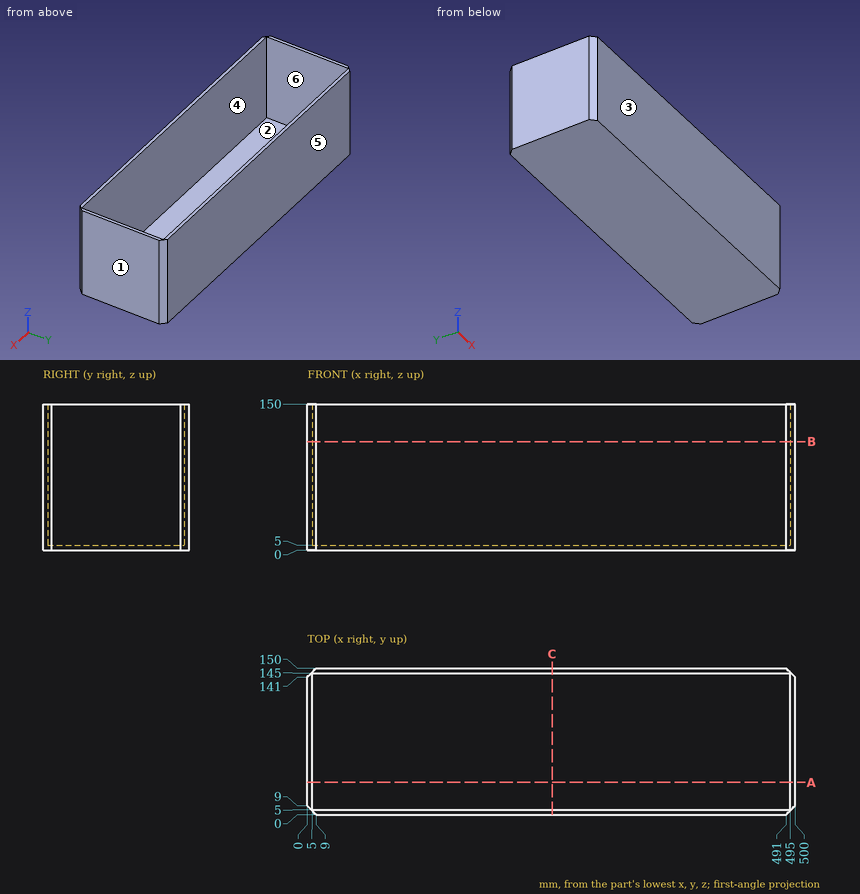
For this review, use the dimensioned drawing (mm, ordinates from the lowest corner) and the shaded views. A direction names the side the tool comes from. Give positions to 0.01 mm unless a question says otherwise; leave off trailing zeros. Order: outer loops, then holes, each group sorted by start corner. A loop starts at its lowest first (then second) coordinate and runs counter-clockwise, first axis right, second up. Notation, with made-up numbers: (-21, 7.25) - (35, 7.25) arc R8 ccw to (35, 13.25) - close; hole circle Ø9 at (-24, 28). An arc over 180 degrees is marked (long way). Use CSV: the item, a comma, the result in double quotes. Start each with the question number.
Q1. To check wall thickness, follow line 1 along Y through (x, z) = (461, 96); line 2 along X through (y, z) = (121, 10); line 3 along Z through (x, y) = (127, 45). State the ranges of each line that lie inside material, in increasing order. Write a range as [from, to].
Q2. We need section A-A, the plane y = 33. Write out the cut boundary in (x, z), and give its area (3 significant figures).
Q3. We need section B-B, the plane z = 111.5. Write out the cut boundary in (x, y).
Q4. We need section C-C, the plane x = 251. Write out the cut boundary in (y, z), and give its area (3 significant figures).
Q5. Clearance check with a flat-ended pin moving along its axis: pin 1 Ø8 at (x, y) = (161.5, 66) entering from +Z. State where the tip first meets the part, or that it passes through.
Q6. The part is to be moulded in two halves that separate along Y. For the marked faces 3, 4, 5 and 6, say which applies: +Y half, -Y half, draft (parallel to the pull), parting line (faces both ways), or undercut.
Q7. Tool access review of the marked faces 1 and 2: name each direction out of +Z, -Z, +X, -X, +Y, -Y from which nothing blocks a thin tool from reaching the whole face with its end or side.
Outcome:
1,line 1,"y = [0, 5], [145, 150]"
1,line 2,"x = [0, 5], [495, 500]"
1,line 3,"z = [0, 5]"
2,outline,"(0, 0) - (500, 0) - (500, 150) - (495, 150) - (495, 5) - (5, 5) - (5, 150) - (0, 150) - close"
2,area,"3,950 mm^2"
3,outline,"(0, 9) - (9, 0) - (491, 0) - (500, 9) - (500, 141) - (491, 150) - (9, 150) - (0, 141) - close; hole (5, 5) - (495, 5) - (495, 145) - (5, 145) - close"
4,outline,"(0, 0) - (150, 0) - (150, 150) - (145, 150) - (145, 5) - (5, 5) - (5, 150) - (0, 150) - close"
4,area,"2,200 mm^2"
5,pin 1,"stops at z = 5"
6,face 3,"-Y half"
6,face 4,"undercut"
6,face 5,"+Y half"
6,face 6,"undercut"
7,face 1,"+Z, -Z, +X, +Y, -Y"
7,face 2,"+Z"
